```python
from build123d import *

# Parameters (mm, degrees)
SKETCH1_W           = 40.89
SKETCH1_H           = 8.5
BOSS_EXTRUDE1_DEPTH = 1.25
SKETCH2_W           = 1.1
SKETCH2_H           = 1.1
CUT_EXTRUDE1_DEPTH  = 42.782826616


with BuildPart() as part:
    # Sketch1 → Boss-Extrude1 (new, symmetric)
    with BuildSketch(Plane.XY):
        with Locations((20.445, 4.25)):
            Rectangle(SKETCH1_W, SKETCH1_H)
    extrude(amount=BOSS_EXTRUDE1_DEPTH, both=True)

    # Sketch2 → Cut-Extrude1 (cut, through all)
    with BuildSketch(Plane.XZ):
        with Locations((3.935, 0)):
            Rectangle(SKETCH2_W, SKETCH2_H)
        with Locations((1.395, 0)):
            Rectangle(SKETCH2_W, SKETCH2_H)
        with Locations((6.475, 0)):
            Rectangle(SKETCH2_W, SKETCH2_H)
        with Locations((9.015, 0)):
            Rectangle(SKETCH2_W, SKETCH2_H)
        with Locations((11.555, 0)):
            Rectangle(SKETCH2_W, SKETCH2_H)
        with Locations((14.095, 0)):
            Rectangle(SKETCH2_W, SKETCH2_H)
        with Locations((16.635, 0)):
            Rectangle(SKETCH2_W, SKETCH2_H)
        with Locations((19.175, 0)):
            Rectangle(SKETCH2_W, SKETCH2_H)
        with Locations((21.715, 0)):
            Rectangle(SKETCH2_W, SKETCH2_H)
        with Locations((24.255, 0)):
            Rectangle(SKETCH2_W, SKETCH2_H)
        with Locations((26.795, 0)):
            Rectangle(SKETCH2_W, SKETCH2_H)
        with Locations((29.335, 0)):
            Rectangle(SKETCH2_W, SKETCH2_H)
        with Locations((31.875, 0)):
            Rectangle(SKETCH2_W, SKETCH2_H)
        with Locations((34.415, 0)):
            Rectangle(SKETCH2_W, SKETCH2_H)
        with Locations((36.955, 0)):
            Rectangle(SKETCH2_W, SKETCH2_H)
        with Locations((39.495, 0)):
            Rectangle(SKETCH2_W, SKETCH2_H)
    extrude(amount=-CUT_EXTRUDE1_DEPTH, mode=Mode.SUBTRACT)


solid = part.part
```
Geometry: final body of the model. Coordinates: model frame, mm. A direction names the side the tool comes from. Round coordinates to 2 decimals unless told otherwise and drop trailing zeros. Use one line per item in the form item = value.
(1) Section A-A on y = 5.5. Count the separate pieces of the cut face and the enclosed holes in it, and give its area (3 significant figures).
Results list:
separate_pieces = 1
enclosed_holes = 16
area = 82.9 mm^2
(2) Draft query along Z for faces 1 (the face through (20, 0, 0)), 2 (the face through (32, 4, 0.55)), 3 (the face through (20, 4, 1.25)). Return one class per face: pulls with the +Z half, pulls with the -Z half, needs draft (parallel to the pull), parting line crosses it, or undercut.
Results list:
face_1 = needs draft
face_2 = undercut
face_3 = pulls with the +Z half
(3) First-contact query: pin 1 Ø0.6 at (y, z) = (2.5, 0) entering from -X. Flat tip, straight axial feed; report the tip coordinate or a pass-through.
Results list:
pin_1 = 0
(4) Access query for faces 4 (the face through (20, 8.5, 0)), 5 (the face through (19.725, 4, 0)). Directions: +Z, -Z, +X, -X, +Y, -Y. A direction counts if a zero-diameter tool reaches every point of the face in a straight line with its end or side. Return the directions, or none.
Results list:
face_4 = +Z, -Z, +X, -X, +Y
face_5 = +Y, -Y
(5) Ray query, probe 1 along Z at (x, y) = (12, 6). Return the intervals inside material, ascending. Write a range as [from, to].
Results list:
probe_1 = [-1.25, -0.55], [0.55, 1.25]
